Build history of the part. All positions in model axes, mm. A direction names the side the tool comes from. Round coordinates to 2 decimals unless told otherwise and drop trailing zeros. Loops run counter-clockwise (first coordinate to the right, second up) from the corner with the lowest first, then second, coordinate; pieces in that order, holes last. Notation, with made-up numbers: M 77,15 L 131,15 A10 ccw 131,28 Z; hole C 66.25,17.5 d2. An arc over 180 degrees is marked long. One line per item, written item: value.
```python
from build123d import *

# Parameters (mm, degrees)
BASE_EXTRUSION_DEPTH = 30
CHANFREIN1_SIZE      = 0.5


with BuildPart() as part:
    # Esquisse1 → Base-Extrusion (new body)
    with BuildSketch(Plane.XY):
        with BuildLine():
            Line((14.991664351, 0.5), (16.992645468, 0.5))
            ThreePointArc((16.992645468, 0.5), (-17, 0), (16.992645468, -0.5))
            Line((16.992645468, -0.5), (14.991664351, -0.5))
            ThreePointArc((14.991664351, -0.5), (14.756961273, -2.689255286), (14.204299838, -4.820566991))
            ThreePointArc((14.204299838, -4.820566991), (14.236067977, -7.118033989), (12.379033495, -8.471099676))
            ThreePointArc((12.379033495, -8.471099676), (-14.401698945, 4.194170658), (14.991664351, 0.5))
        make_face()
    extrude(amount=BASE_EXTRUSION_DEPTH)

    # Chanfrein1
    chanfrein1_edges = [part.edges().sort_by_distance(p)[0] for p in [
        (-14.401698945, 4.194170658, 30),
        (-17, 0, 30),
        (-17, 0, 0),
        (-14.401698945, 4.194170658, 0),
    ]]
    chamfer(chanfrein1_edges, length=CHANFREIN1_SIZE)


solid = part.part
```
Item 1: Which spindle directions (+Z, -Z, +X, -X, +Y, -Y) get a long thin tool onto all of the face, cutting with end or side? Do faces 4 (the face through (-14.76, 3.36, 0.36)), 5 (the face through (16, -0.5, 15)), 6 (the face through (14.762, -2.659, 14.79)). Say none if no direction does.
Check values:
face 4: -Z
face 5: +Z, -Z, +X
face 6: +Z, -Z
Item 2: Wall check: line 1 along Y through (x, z) = (0, 18.5); line 2 along X through (y, z) = (7, 19); line 3 along X through (y, z) = (13.5, 23.5). Give the ranges that are in metal, low to high.
Check values:
line 1: y = -17 to -15, 15 to 17
line 2: x = -15.49 to -13.27, 13.27 to 15.49
line 3: x = -10.33 to -6.54, 6.54 to 10.33
Item 3: Drop flat-ended pins along their axis: P1, Ø2, axis at x = 16, z = 16, coming from the +Y side; P2, Ø1.5, axis at y = 5.5, z = 26, coming from the +X side; P3, Ø2, axis at x = 16.5, z = 11, coming from the -Y side. Give the stop position or say it passes through.
Check values:
P1: stops at y = 8
P2: stops at x = 16.32
P3: stops at y = -6.98
Item 4: Slice it at C-C, the plane z = 25. Give the cut face in (x, y), and give its area (3 significant figures).
Check values:
outline: M 12.38,-8.47 A15 cw long 14.99,0.5 L 16.99,0.5 A17 ccw long 16.99,-0.5 L 14.99,-0.5 A15 cw 14.2,-4.82 A2.5 cw Z
area: 196 mm2
Item 5: Slice it at A-A, the plane x = 0. Give the cut face in (y, z).
Check values:
outline: M -17,0.5 L -16.5,0 L -15.5,0 L -15,0.5 L -15,29.5 L -15.5,30 L -16.5,30 L -17,29.5 Z; M 15,0.5 L 15.5,0 L 16.5,0 L 17,0.5 L 17,29.5 L 16.5,30 L 15.5,30 L 15,29.5 Z
Item 6: Slice it at B-B, the plane y = 0. Give the cut face in (x, z), and give its area (3 significant figures).
Check values:
outline: M -17,0.5 L -16.5,0 L -15.5,0 L -15,0.5 L -15,29.5 L -15.5,30 L -16.5,30 L -17,29.5 Z
area: 59.5 mm2
Item 7: Pull direction Y, two halves, no side cores. Call faces 1 (the face through (15, -4, 30)), 2 (the face through (-16.984, 0.74, 14.797)), 3 (the face through (-14.76, 3.36, 29.64)): pulls with the +Y half, pulls with the -Y half, needs draft (parallel to the pull), parting line crosses it, or undercut.
Check values:
face 1: needs draft
face 2: parting line crosses it
face 3: undercut
